from build123d import *

# Parameters (mm, degrees)
SKETCH1_W           = 100
SKETCH1_H           = 20
BOSS_EXTRUDE1_DEPTH = 6
SKETCH2_W           = 100
SKETCH2_H           = 20
CUT_EXTRUDE3_DEPTH  = 3
BOSS_EXTRUDE2_DEPTH = 72
SHELL1_START        = 2
SHELL1_DEPTH        = 74
SHELL1_START_2      = 5
SHELL1_2_DEPTH      = 71
CUT_EXTRUDE4_START  = -72
CUT_EXTRUDE4_DEPTH  = 72
BOSS_EXTRUDE3_DEPTH = 6


# Read off the part's stored shape, not the designer's step: Shell1
with BuildPart() as part:
    # Sketch1 → Boss-Extrude1 (new body)
    with BuildSketch(Plane(origin=(0, 0, 0), x_dir=(1, 0, 0), z_dir=(0, 1, 0))):
        with BuildLine():
            Line((-50, 141.421356237), (-50, 50))
            Line((-50, 50), (50, 50))
            Line((50, 50), (50, 141.421356237))
            ThreePointArc((50, 141.421356237), (0, 150), (-50, 141.421356237))
        make_face()
        with BuildLine():
            Line((-70, 50), (-50, 50))
            Line((-50, 50), (-50, 141.421356237))
            ThreePointArc((-50, 141.421356237), (-60.159525267, 137.407538074), (-70, 132.664991614))
            Line((-70, 132.664991614), (-70, 50))
        make_face()
        with Locations((0, 40)):
            Rectangle(SKETCH1_W, SKETCH1_H)
        with BuildLine():
            Line((50, 141.421356237), (50, 50))
            Line((50, 50), (70, 50))
            Line((70, 50), (70, 132.664991614))
            ThreePointArc((70, 132.664991614), (60.159525267, 137.407538074), (50, 141.421356237))
        make_face()
    extrude(amount=BOSS_EXTRUDE1_DEPTH)

    # Sketch2 → Cut-Extrude3 (cut)
    with BuildSketch(Plane.XZ):
        with BuildLine():
            ThreePointArc((-70, -132.664991614), (-60.159525267, -137.407538074), (-50, -141.421356237))
            Line((-50, -141.421356237), (-50, -50))
            Line((-50, -50), (-70, -50))
            Line((-70, -50), (-70, -132.664991614))
        make_face()
        with Locations((0, -40)):
            Rectangle(SKETCH2_W, SKETCH2_H)
        with BuildLine():
            Line((50, -50), (50, -141.421356237))
            ThreePointArc((50, -141.421356237), (60.159525267, -137.407538074), (70, -132.664991614))
            Line((70, -132.664991614), (70, -50))
            Line((70, -50), (50, -50))
        make_face()
    extrude(amount=-CUT_EXTRUDE3_DEPTH, mode=Mode.SUBTRACT)

    # Sketch3 → Boss-Extrude2 (add)
    with BuildSketch(Plane(origin=(0, 6, 0), x_dir=(-1, 0, 0), z_dir=(0, 1, 0))):
        with BuildLine():
            Line((50, -50), (-50, -50))
            Line((-50, -50), (-50, -141.421356237))
            ThreePointArc((-50, -141.421356237), (0, -150), (50, -141.421356237))
            Line((50, -141.421356237), (50, -50))
        make_face()
    extrude(amount=BOSS_EXTRUDE2_DEPTH)

    # Shell1 outline → Shell1 (cut)
    with BuildSketch(Plane(origin=(0, 0, 0), x_dir=(1, 0, 0), z_dir=(0, 1, 0)).offset(SHELL1_START)):
        with BuildLine():
            Line((48, 52), (48, 140))
            ThreePointArc((48, 140), (0, 148), (-48, 140))
            Line((-48, 140), (-48, 52))
            Line((-48, 52), (48, 52))
        make_face()
    extrude(amount=SHELL1_DEPTH, mode=Mode.SUBTRACT)

    # Shell1 2 outline → Shell1 2 (cut)
    with BuildSketch(Plane(origin=(0, 0, 0), x_dir=(1, 0, 0), z_dir=(0, 1, 0)).offset(SHELL1_START_2)):
        with BuildLine():
            Line((50, 52), (50, 139.298241195))
            ThreePointArc((50, 139.298241195), (49.001256273, 139.652700954), (48, 140))
            Line((48, 140), (48, 52))
            Line((48, 52), (50, 52))
        make_face()
    extrude(amount=SHELL1_2_DEPTH, mode=Mode.SUBTRACT)

    # Sketch4 → Cut-Extrude4 (cut)
    with BuildSketch(Plane(origin=(0, 78, 0), x_dir=(-1, 0, 0), z_dir=(0, 1, 0)).offset(CUT_EXTRUDE4_START)):
        with BuildLine():
            Line((50, -52), (-50, -52))
            Line((-50, -52), (-50, -139.298241195))
            ThreePointArc((-50, -139.298241195), (0, -148), (50, -139.298241195))
            Line((50, -139.298241195), (50, -52))
        make_face()
    extrude(amount=CUT_EXTRUDE4_DEPTH, mode=Mode.SUBTRACT)

    # Sketch5 → Boss-Extrude3 (add)
    with BuildSketch(Plane.XZ):
        with BuildLine():
            Line((-50, -141.421356237), (-50, -50))
            Line((-50, -50), (50, -50))
            Line((50, -50), (50, -141.421356237))
            ThreePointArc((50, -141.421356237), (0, -150), (-50, -141.421356237))
        make_face()
    extrude(amount=-BOSS_EXTRUDE3_DEPTH)


solid = part.part
Here's how the part is built. I have some questions about the finished solid (model axes, mm). A direction names the side the tool comes from. Round coordinates to 2 decimals unless told otherwise and drop trailing zeros. Order: outer loops, then holes, each group sorted by start corner. A loop starts at its lowest first (then second) coordinate and runs counter-clockwise, first axis right, second up. Notation, with made-up numbers: M 70,-34.5 L 80,-34.5 A28 ccw 80,-10.5 Z; hole C -33,31 d3. An arc over 180 degrees is marked long. Return JSON: item names as keys, results as strings. Group by question number.
1. If we section it at A-A on y = 54: List the corners of the cut face in (x, z) for me.
2. If we section it at D-D on x = 6: List the corners of the cut face in (y, z) for me.
3. On a 3-axis mill with a long thin cutter (end or side, diameter ignored), from which of +Z, -Z, +X, -X, +Y, -Y can I reach the whole of each face in a straight line? I mean faces 1 (the face through (-1, 3, -40)), 2 (the face through (-60, 3, -95)), 3 (the face through (60, 3, -95)), 4 (the face through (-1, 41, -50)), 5 (the face through (-1, 41, -52)). Say none if no direction works.
4. If we section it at C-C on x = -20.5: List the corners of the cut face in (y, z) for me.
5. Please list where these lines run through material, in increasing order: probe 1 along Z at (x, y) = (2, 14.5); probe 2 along Y at (x, z) = (-14, -48.5); probe 3 along Z at (x, y) = (27, 20.5).
6. I'm going to push flat-ended pins straight in: pin 1 Ø1.5 at (x, y) = (-37, 66) entering from -Z; pin 2 Ø10 at (x, z) = (22.5, -57.5) entering from +Y; pin 3 Ø10 at (x, z) = (56, -82.5) entering from -Y; pin 4 Ø4 at (y, z) = (51.5, -136) entering from -X. Where does each tip first touch, or does it pass through?
7. If we section it at B-B on z = -70.5: List the corners of the cut face in (x, y) for me, then the cut area to 3 significant figures.
Reply:
{
 "1": {"outline": "M -50,-141.42 A150 ccw 50,-141.42 L 50,-139.3 A148 cw 48,-140 A148 cw -50,-139.3 Z; M -50,-52 L 50,-52 L 50,-50 L -50,-50 Z"},
 "2": {"outline": "M 0,-149.88 L 78,-149.88 L 78,-147.88 L 6,-147.88 L 6,-52 L 78,-52 L 78,-50 L 6,-50 L 6,-30 L 3,-30 L 3,-50 L 0,-50 Z"},
 "3": {"face 1": "+Z, +X, -X, -Y", "face 2": "+Z, -Z, -X, -Y", "face 3": "+Z, -Z, +X, -Y", "face 4": "+Z, +X, -X, +Y", "face 5": "+X, -X, +Y"},
 "4": {"outline": "M 0,-148.59 L 78,-148.59 L 78,-146.57 L 6,-146.57 L 6,-52 L 78,-52 L 78,-50 L 6,-50 L 6,-30 L 3,-30 L 3,-50 L 0,-50 Z"},
 "5": {"probe 1": "-149.99 to -147.99, -52 to -50", "probe 2": "3 to 6", "probe 3": "-147.55 to -145.52, -52 to -50"},
 "6": {"pin 1": "z = -145.55", "pin 2": "y = 6", "pin 3": "y = 3", "pin 4": "through"},
 "7": {"outline": "M -70,3 L -50,3 L -50,0 L 50,0 L 50,3 L 70,3 L 70,6 L -70,6 Z", "area": "720 mm^2"}
}
